Check sheet for the modelled part. Datum: model origin and axes. Units: mm. A direction names the side the tool comes from. Round coordinates to 2 decimals unless told otherwise and drop trailing zeros. Order: outer loops, then holes, each group sorted by start corner. A loop starts at its lowest first (then second) coordinate and runs counter-clockwise, first axis right, second up.
(1) Sectioned sample at A-A, the plane x = 22. Enter the section's corners in (y, z) (3 decimals), and give its area (3 significant figures).
(2) Mould release check, pull along X, two halves, no side actions. Record for faces 1 (the cylindrical face through (-10.45, 10.14, 5.43)), 2 (the flat face through (29.91, 17.57, 18.77)), 3 (the cylindrical face through (24.43, 1.97, 34.4)): released by +X, released by -X, zero draft, split by the parting line, or undercut.
(3) Sectioned sample at C-C, the plane z = 16. Enter the section's corners in (x, y).
(4) Tool access check on faces 4 (the cylindrical face through (24.55, 10.14, 5.43)), 5 (the flat face through (-17.6, 10, 3)), 6 (the flat face through (0, 9, 41)), 7 (the flat face through (12.2, 3.8, 39.175)), 8 (the flat face through (44, 10, 5)). Record the directions out of +Z, -Z, +X, -X, +Y, -Y that give a thin tool (end or side, any length) a straight path to the whole face; none if there is none.
(5) Depth check by flat-ended pin: pin 1 (6 mm diameter, centred on y = 10.5, z = 16, fed in from -X); pin 2 (12 mm diameter, centred on y = 7, z = 13.5, fed in from +X); pin 3 (1.6 mm diameter, centred on x = 17.5, z = 38.5, fed in from +Y). Enter the tip coordinate at first touch or a pass-through.
(6) Sectioned sample at D-D, the plane x = -15. Enter the section's corners in (y, z), and give its area (3 significant figures).
(7) Sectioned sample at B-B, the plane y = 10.5. Count the separate pieces of the cut face and the enclosed holes in it, and give its area (3 significant figures).
(8) Thickness scan on probe 1 along X at (y, z) = (11, 4); probe 2 along X at (y, z) = (9.25, 14.5); probe 3 along Z at (x, y) = (21, 11.25). Record the ranges inside material, lowest first.
```python
from build123d import *

# Parameters (mm, degrees)
BOSS_EXTRUDE1_DEPTH = 35
CUT_EXTRUDE1_DEPTH  = 25
SKETCH3_W           = 25
SKETCH3_H           = 28.356409098
BOSS_EXTRUDE2_DEPTH = 5
BOSS_EXTRUDE3_DEPTH = 10
SKETCH5_W           = 28.356409098
SKETCH5_H           = 20
BOSS_EXTRUDE4_DEPTH = 10
SKETCH6_W           = 55
SKETCH6_H           = 15
BOSS_EXTRUDE5_DEPTH = 9.818590902
SKETCH7_W           = 28.356409098
SKETCH7_H           = 20
BOSS_EXTRUDE6_DEPTH = 10
SKETCH8_W           = 65
SKETCH8_H           = 20
BOSS_EXTRUDE7_DEPTH = 5
SKETCH9_W           = 10
SKETCH9_H           = 20
CUT_EXTRUDE2_DEPTH  = 28.356409098
SKETCH10_W          = 9.818590902
SKETCH10_H          = 15
CUT_EXTRUDE3_DEPTH  = 10
SKETCH11_W          = 10
SKETCH11_H          = 20
CUT_EXTRUDE4_DEPTH  = 28.356409098
SKETCH12_W          = 15
SKETCH12_H          = 1.643590902
CUT_EXTRUDE5_DEPTH  = 25
SKETCH13_W          = 25
SKETCH13_H          = 20
CUT_EXTRUDE6_DEPTH  = 28.356409098
CUT_EXTRUDE7_REACH  = 64.926
SKETCH14_W          = 25
SKETCH14_H          = 11
SKETCH15_W          = 25
SKETCH15_H          = 3.175
CUT_EXTRUDE8_DEPTH  = 1
CUT_EXTRUDE9_REACH  = 72.854
SKETCH16_W          = 3.175
SKETCH16_H          = 12
CUT_EXTRUDE10_REACH = 72.854
SKETCH17_W          = 12
SKETCH17_H          = 3.175
CUT_EXTRUDE11_REACH = 67.491
SKETCH18_W          = 25
SKETCH18_H          = 11
CUT_EXTRUDE12_DEPTH = 66.491072865
CUT_EXTRUDE13_DEPTH = 63.308351166
FILLET1_R           = 1.5
FILLET2_R           = 2
FILLET3_R           = 5


with BuildPart() as part:
    # Boss-Extrude1: read off the stored shape, not the designer's step
    # Boss-Extrude1 outline → Boss-Extrude1 (new body)
    with BuildSketch(Plane.YZ):
        Polygon((0, 5), (20, 5), (15, 33.356409098), (0, 33.356409098), align=None)
    extrude(amount=BOSS_EXTRUDE1_DEPTH)

    # Sketch2 → Cut-Extrude1 (cut)
    with BuildSketch(Plane.ZY):
        Polygon((33.356409098, 15), (5, 20), (5, 15), align=None)
    extrude(amount=-CUT_EXTRUDE1_DEPTH, mode=Mode.SUBTRACT)

    # Sketch3 → Boss-Extrude2 (add)
    with BuildSketch(Plane(origin=(0, 15, 0), x_dir=(-1, 0, 0), z_dir=(0, 1, 0))):
        with Locations((-12.5, 19.178204549)):
            Rectangle(SKETCH3_W, SKETCH3_H)
    extrude(amount=BOSS_EXTRUDE2_DEPTH)

    # Sketch4 → Boss-Extrude3 (add)
    with BuildSketch(Plane.ZY):
        Polygon((5, 20), (33.356409098, 15), (33.356409098, 0), (5, 0), align=None)
    extrude(amount=BOSS_EXTRUDE3_DEPTH)

    # Sketch5 → Boss-Extrude4 (add)
    with BuildSketch(Plane.ZY.offset(10)):
        with Locations((19.178204549, 10)):
            Rectangle(SKETCH5_W, SKETCH5_H)
    extrude(amount=BOSS_EXTRUDE4_DEPTH)

    # Sketch6 → Boss-Extrude5 (add)
    with BuildSketch(Plane.XY.offset(33.356409098)):
        with Locations((7.5, 7.5)):
            Rectangle(SKETCH6_W, SKETCH6_H)
    extrude(amount=BOSS_EXTRUDE5_DEPTH)

    # Sketch7 → Boss-Extrude6 (add)
    with BuildSketch(Plane(origin=(35, 0, 0), x_dir=(0, 0, -1), z_dir=(1, 0, 0))):
        with Locations((-19.178204549, 10)):
            Rectangle(SKETCH7_W, SKETCH7_H)
    extrude(amount=BOSS_EXTRUDE6_DEPTH)

    # Sketch8 → Boss-Extrude7 (add)
    with BuildSketch(Plane(origin=(0, 0, 5), x_dir=(-1, 0, 0), z_dir=(0, 0, -1))):
        with Locations((-12.5, 10)):
            Rectangle(SKETCH8_W, SKETCH8_H)
    extrude(amount=BOSS_EXTRUDE7_DEPTH)

    # Sketch9 → Cut-Extrude2 (cut)
    with BuildSketch(Plane.XY.offset(33.356409098)):
        with Locations((40, 10)):
            Rectangle(SKETCH9_W, SKETCH9_H)
    extrude(amount=-CUT_EXTRUDE2_DEPTH, mode=Mode.SUBTRACT)

    # Sketch10 → Cut-Extrude3 (cut)
    with BuildSketch(Plane.ZY.offset(20)):
        with Locations((38.265704549, 7.5)):
            Rectangle(SKETCH10_W, SKETCH10_H)
    extrude(amount=-CUT_EXTRUDE3_DEPTH, mode=Mode.SUBTRACT)

    # Sketch11 → Cut-Extrude4 (cut)
    with BuildSketch(Plane.XY.offset(33.356409098)):
        with Locations((-15, 10)):
            Rectangle(SKETCH11_W, SKETCH11_H)
    extrude(amount=-CUT_EXTRUDE4_DEPTH, mode=Mode.SUBTRACT)

    # Sketch12 → Cut-Extrude5 (cut)
    with BuildSketch(Plane(origin=(0, 0, 0), x_dir=(0, -1, 0), z_dir=(-1, 0, 0))):
        with Locations((-7.5, 34.178204549)):
            Rectangle(SKETCH12_W, SKETCH12_H)
    extrude(amount=-CUT_EXTRUDE5_DEPTH, mode=Mode.SUBTRACT)

    # Sketch13 → Cut-Extrude6 (cut)
    with BuildSketch(Plane.XY.offset(33.356409098)):
        with Locations((12.5, 10)):
            Rectangle(SKETCH13_W, SKETCH13_H)
    extrude(amount=-CUT_EXTRUDE6_DEPTH, mode=Mode.SUBTRACT)

    # Sketch14 → Cut-Extrude7 (cut, up to next)
    with BuildSketch(Plane.XY.offset(39.175), mode=Mode.PRIVATE) as cut_extrude7_sk1:
        with Locations((12.5, 9.5)):
            Rectangle(SKETCH14_W, SKETCH14_H)
    cut_extrude7_tool1 = extrude(cut_extrude7_sk1.sketch, amount=-CUT_EXTRUDE7_REACH, mode=Mode.PRIVATE) & part.part
    add(cut_extrude7_tool1.solids().sort_by_distance((12.5, 9.5, 39.175))[0], mode=Mode.SUBTRACT)

    # Sketch15 → Cut-Extrude8 (cut)
    with BuildSketch(Plane(origin=(0, 4, 0), x_dir=(-1, 0, 0), z_dir=(0, 1, 0))):
        with Locations((-12.5, 37.5875)):
            Rectangle(SKETCH15_W, SKETCH15_H)
    extrude(amount=-CUT_EXTRUDE8_DEPTH, mode=Mode.SUBTRACT)

    # Sketch16 → Cut-Extrude9 (cut, up to next)
    with BuildSketch(Plane(origin=(32.5, 0, 0), x_dir=(0, 0, -1), z_dir=(1, 0, 0)), mode=Mode.PRIVATE) as cut_extrude9_sk1:
        with Locations((-37.5875, 9)):
            Rectangle(SKETCH16_W, SKETCH16_H)
    cut_extrude9_tool1 = extrude(cut_extrude9_sk1.sketch, amount=-CUT_EXTRUDE9_REACH, mode=Mode.PRIVATE) & part.part
    add(cut_extrude9_tool1.solids().sort_by_distance((32.5, 9, 37.5875))[0], mode=Mode.SUBTRACT)

    # Sketch17 → Cut-Extrude10 (cut, up to next)
    with BuildSketch(Plane(origin=(-7.5, 0, 0), x_dir=(0, -1, 0), z_dir=(-1, 0, 0)), mode=Mode.PRIVATE) as cut_extrude10_sk1:
        with Locations((-9, 37.5875)):
            Rectangle(SKETCH17_W, SKETCH17_H)
    cut_extrude10_tool1 = extrude(cut_extrude10_sk1.sketch, amount=-CUT_EXTRUDE10_REACH, mode=Mode.PRIVATE) & part.part
    add(cut_extrude10_tool1.solids().sort_by_distance((-7.5, 9, 37.5875))[0], mode=Mode.SUBTRACT)

    # Sketch18 → Cut-Extrude11 (cut, up to next)
    with BuildSketch(Plane.XY.offset(43.175), mode=Mode.PRIVATE) as cut_extrude11_sk1:
        with Locations((12.5, 9.5)):
            Rectangle(SKETCH18_W, SKETCH18_H)
    cut_extrude11_tool1 = extrude(cut_extrude11_sk1.sketch, amount=-CUT_EXTRUDE11_REACH, mode=Mode.PRIVATE) & part.part
    add(cut_extrude11_tool1.solids().sort_by_distance((12.5, 9.5, 43.175))[0], mode=Mode.SUBTRACT)

    # Sketch19 → Cut-Extrude12 (cut, through all)
    with BuildSketch(Plane(origin=(0, 0, 0), x_dir=(-1, 0, 0), z_dir=(0, 0, -1))):
        with BuildLine():
            Line((-37.4, 7.5), (-37.4, 12.5))
            ThreePointArc((-37.4, 12.5), (-40, 15.1), (-42.6, 12.5))
            Line((-42.6, 12.5), (-42.6, 7.5))
            ThreePointArc((-42.6, 7.5), (-40, 4.9), (-37.4, 7.5))
        make_face()
    extrude(amount=-CUT_EXTRUDE12_DEPTH, mode=Mode.SUBTRACT)

    # Sketch20 → Cut-Extrude13 (cut, through all)
    with BuildSketch(Plane.XY.offset(5)):
        with BuildLine():
            Line((-12.4, 7.5), (-12.4, 12.5))
            ThreePointArc((-12.4, 12.5), (-15, 15.1), (-17.6, 12.5))
            Line((-17.6, 12.5), (-17.6, 7.5))
            ThreePointArc((-17.6, 7.5), (-15, 4.9), (-12.4, 7.5))
        make_face()
    extrude(amount=-CUT_EXTRUDE13_DEPTH, mode=Mode.SUBTRACT)

    # Fillet1
    fillet1_edges = [part.edges().sort_by_distance(p)[0] for p in [
        (35, 10, 5),
        (-10, 10, 5),
        (0, 10, 5),
        (25, 10, 5),
    ]]
    fillet(fillet1_edges, radius=FILLET1_R)

    # Fillet2
    fillet2_edges = [part.edges().sort_by_distance(p)[0] for p in [
        (-20, 0, 2.5),
        (0, 2, 35),
        (45, 0, 2.5),
        (45, 20, 2.5),
        (25, 2, 35),
        (-20, 20, 2.5),
        (-10, 7.5, 43.175),
        (35, 7.5, 43.175),
    ]]
    fillet(fillet2_edges, radius=FILLET2_R)

    # Fillet3
    fillet3_edges = [part.edges().sort_by_distance(p)[0] for p in [
        (30, 15, 33.356409098),
        (-5, 15, 33.356409098),
    ]]
    fillet(fillet3_edges, radius=FILLET3_R)


solid = part.part
```
Derived:
1. outline: (0, 0) - (20, 0) - (20, 5) - (0, 5) - close; (0, 35) - (4, 35) - (4, 36) - (3, 36) - (3, 39.175) - (4, 39.175) - (4, 43.175) - (0, 43.175) - close
1. area: 130 mm2
2. face 1: released by -X
2. face 2: zero draft
2. face 3: undercut
3. outline: (-10, 0) - (0, 0) - (0, 18.06) - (-10, 18.06) - close; (25, 0) - (35, 0) - (35, 18.06) - (25, 18.06) - close
4. face 4: +Y, -Y
4. face 5: +Z, -Z
4. face 6: +Z, +Y
4. face 7: +Y
4. face 8: +Z, +X, +Y, -Y
5. pin 1: stops at x = -10
5. pin 2: stops at x = 35
5. pin 3: stops at y = 4
6. outline: (0, 0) - (4.9, 0) - (4.9, 5) - (0, 5) - close; (15.1, 0) - (20, 0) - (20, 5) - (15.1, 5) - close
6. area: 49.0 mm2
7. separate pieces: 3
7. enclosed holes: 0
7. area: 989 mm2
8. probe 1: x = -20 to -17.6, -12.4 to 37.4, 42.6 to 45
8. probe 2: x = -10 to 0, 25 to 35
8. probe 3: z = 0 to 5
